from build123d import *

# Parameters (mm, degrees)
SKETCH1_W            = 40
SKETCH1_H            = 50
BOSS_EXTRUDE1_DEPTH  = 6.54
M4_CLEARANCE_HOLE1_D = 4.5
CUT_EXTRUDE1_DEPTH   = 33.676774627


with BuildPart() as part:
    # Sketch1 → Boss-Extrude1 (new body)
    with BuildSketch(Plane.XY):
        Rectangle(SKETCH1_W, SKETCH1_H)
    extrude(amount=BOSS_EXTRUDE1_DEPTH)

    # M4 Clearance Hole1 (through all)
    with Locations(Plane(origin=(0, 0, 0), x_dir=(-1, 0, 0), z_dir=(0, 0, -1))):
        with Locations((-12.5, 15.5), (12.5, 15.5), (12.5, -15.5), (-12.5, -15.5)):
            Hole(M4_CLEARANCE_HOLE1_D / 2)

    # Sketch6 → Cut-Extrude1 (cut, through all)
    with BuildSketch(Plane(origin=(0, 0, 0), x_dir=(-1, 0, 0), z_dir=(0, 0, -1))):
        Polygon((20, 16.996094703), (20, -16.996094703), (6.403124237, 0), align=None)
        Polygon((13.596875763, -25), (-13.596875763, -25), (0, -8.003905297), align=None)
        Polygon((-20, 16.996094703), (-20, -16.996094703), (-6.403124237, 0), align=None)
        Polygon((-13.596875763, 25), (13.596875763, 25), (0, 8.003905297), align=None)
    extrude(amount=-CUT_EXTRUDE1_DEPTH, mode=Mode.SUBTRACT)


solid = part.part
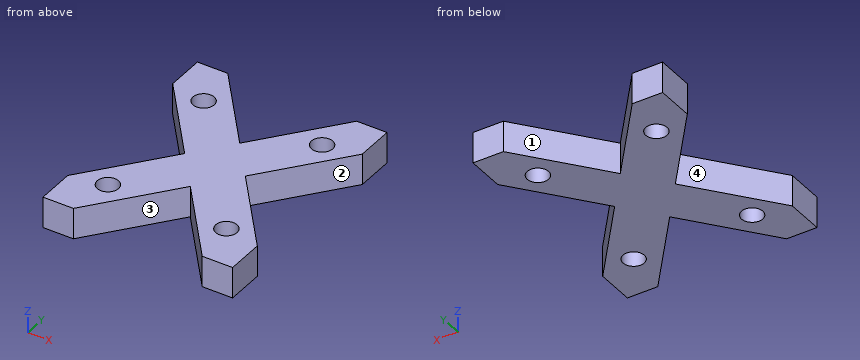
Geometry check sheet. Reference: the model listing, model coordinates, mm. Face numbers are marked on the shaded views. Give positions to 0.01 mm unless a question says otherwise; leave off trailing zeros. Write each loop counter-clockwise with the first axis right and the second up, starting at its lowest first coordinate (ties: lowest second). Pieces come first, ordered by that corner, then holes. Notation, with made-up numbers: M 36,24.5 L 54,24.5 A6 cw 54,29.5 Z; hole C 5,-13.75 d11. An arc over 180 degrees is marked long. Answer as CSV lines item,"result". Start each with the question number.
Q1. Material ranges on L1, parallel to Y at x = -13, z = 0.75; L2, parallel to Y at x = 12.5, z = 1.5; L3, parallel to X at y = 14, z = 6.5, recorded low to high.
Q2. Release check for a two-part mould opening along Y. For the marked faces 1, 2, 3 and 4 record: pulls with the +Y half, pulls with the -Y half, needs draft (parallel to the pull), parting line crosses it, or undercut.
Q3. Section check B-B, the plane y = -18.5. Record the cut outline in (x, z), then the cut area to 3 significant figures.
Q4. Go/stop test with flat-tipped pins: pin 1 (1.5 mm diameter, centred on x = -8.5, z = 2.5, fed in from +Y); pin 2 (2 mm diameter, centred on x = 11, z = 1.5, fed in from -Y); pin 3 (1.5 mm diameter, centred on x = -5, z = 3.5, fed in from -Y). Record where each tip stops, or that it passes through.
Q5. Section check A-A, the plane z = 2.5. Record the cut outline in (x, y), then the cut area to 3 significant figures.
Q6. Section check D-D, the plane x = 11.5. Record the cut outline in (y, z), then the cut area to 3 significant figures.
Q7. Section check C-C, the plane x = -17. Record the cut outline in (y, z), then the cut area to 3 significant figures.
Geometry says:
1,L1,"-24.25 to -17.69, -13.31 to -8.25, 8.25 to 13.31, 17.69 to 24.25"
1,L2,"-23.63 to -17.75, -13.25 to -7.62, 7.62 to 13.25, 17.75 to 23.63"
1,L3,"-17.6 to -14.18, -10.82 to -4.8, 4.8 to 10.82, 14.18 to 17.6"
2,face 1,"pulls with the +Y half"
2,face 2,"undercut"
2,face 3,"pulls with the -Y half"
2,face 4,"undercut"
3,outline,"M -20,0 L -8.4,0 L -8.4,6.54 L -20,6.54 Z; M 8.4,0 L 20,0 L 20,6.54 L 8.4,6.54 Z"
3,area,"152 mm^2"
4,pin 1,"y = 19.57"
4,pin 2,"y = -23"
4,pin 3,"y = -15.19"
5,outline,"M -20,-25 L -13.6,-25 L 0,-8 L 13.6,-25 L 20,-25 L 20,-17 L 6.4,0 L 20,17 L 20,25 L 13.6,25 L 0,8 L -13.6,25 L -20,25 L -20,17 L -6.4,0 L -20,-17 Z; hole C -12.5,-15.5 d4.5; hole C -12.5,15.5 d4.5; hole C 12.5,-15.5 d4.5; hole C 12.5,15.5 d4.5"
5,area,"1,010 mm^2"
6,outline,"M -22.38,0 L -17.52,0 L -17.52,6.54 L -22.38,6.54 Z; M -13.48,0 L -6.37,0 L -6.37,6.54 L -13.48,6.54 Z; M 6.37,0 L 13.48,0 L 13.48,6.54 L 6.37,6.54 Z; M 17.52,0 L 22.38,0 L 22.38,6.54 L 17.52,6.54 Z"
6,area,"157 mm^2"
7,outline,"M -25,0 L -13.25,0 L -13.25,6.54 L -25,6.54 Z; M 13.25,0 L 25,0 L 25,6.54 L 13.25,6.54 Z"
7,area,"154 mm^2"
